```python
from build123d import *

# Parameters (mm, degrees)
BOSS_EXTRUDE2_DEPTH = 76.2


with BuildPart() as part:
    # Sketch4 → Boss-Extrude2 (new body)
    with BuildSketch(Plane(origin=(0, 0, 0), x_dir=(0, 0, -1), z_dir=(1, 0, 0))):
        Polygon((0, 0), (0, 20.6375), (-38.1, 20.6375), (-38.1, 14.2875), (-6.35, 14.2875), (-6.35, 0), align=None)
        Polygon((0, -20.6375), (0, 0), (-6.35, 0), (-6.35, -14.2875), (-38.1, -14.2875), (-38.1, -20.6375), align=None)
    extrude(amount=BOSS_EXTRUDE2_DEPTH)


solid = part.part
```
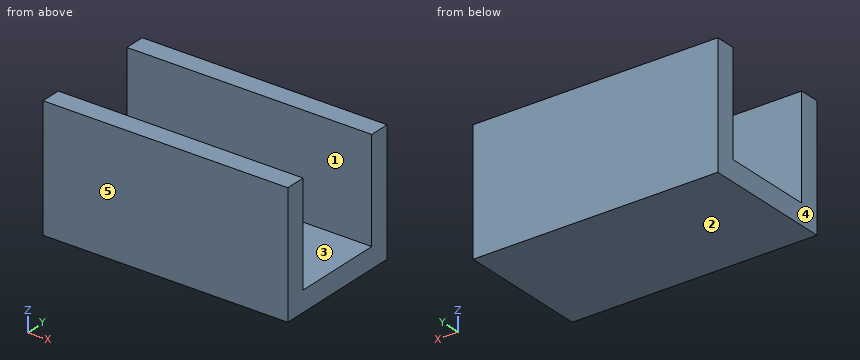
Read the model definition and answer for the solid it produces. Units are mm, in the model's axes. Face numbers are marked on the shaded views. A direction names the side the tool comes from. Round coordinates to 2 decimals unless told otherwise and drop trailing zeros. Write each loop counter-clockwise with the first axis right and the second up, starting at its lowest first coordinate (ties: lowest second). Pieces come first, ordered by that corner, then holes. Notation, with made-up numbers: (4, -27) - (37, -27) arc R13 ccw to (37, -15) - close; hole circle Ø3 at (17, -5.75). An arc over 180 degrees is marked (long way). One line per item, written item: value.
Q1. Find section A-A (z = 22). Determine the outline of the cut face in (x, y), and give its area (3 significant figures).
The answers:
outline: (0, -20.64) - (76.2, -20.64) - (76.2, -14.29) - (0, -14.29) - close; (0, 14.29) - (76.2, 14.29) - (76.2, 20.64) - (0, 20.64) - close
area: 968 mm2
Q2. For a pull along Y with two mould halves and no side action, classify the marked faces 3, 4 and 5 as pulls with the +Y half, pulls with the -Y half, needs draft (parallel to the pull), parting line crosses it, or undercut.
The answers:
face 3: undercut
face 4: needs draft
face 5: pulls with the -Y half
Q3. This flat-tipped pin is pushed along its axis until it touches: P1, Ø23, axis at x = 32.5, y = -2, coming from the +Z side. Where does it stop, or does it pass through?
The answers:
P1: stops at z = 6.35
Q4. Which of the six approach directions +Z, -Z, +X, -X, +Y, -Y give full straight-line access (tool end or side, diameter ignored) to the marked faces 1 and 2?
The answers:
face 1: +Z, +X, -X
face 2: -Z, +X, -X, +Y, -Y
Q5. Find section C-C (y = -7). Determine the outline of the cut face in (x, z), and give its area (3 significant figures).
The answers:
outline: (0, 0) - (76.2, 0) - (76.2, 6.35) - (0, 6.35) - close
area: 484 mm2
Q6. Find section B-B (x = 66.5). Determine the outline of the cut face in (y, z), and give its area (3 significant figures).
The answers:
outline: (-20.64, 0) - (20.64, 0) - (20.64, 38.1) - (14.29, 38.1) - (14.29, 6.35) - (-14.29, 6.35) - (-14.29, 38.1) - (-20.64, 38.1) - close
area: 665 mm2
Q7. Straight lines are drawn through the part: line 1 (Y direction, x = 60.5, z = 32); line 2 (Z direction, x = 12, y = 12). For each, find the intervals that lie inside material, in ascending order. Write a range as from..to.
The answers:
line 1: y = -20.64..-14.29, 14.29..20.64
line 2: z = 0..6.35
